Drawing for the job (mm, zero at the part's lowest x, y, z). Give positions to 0.01 mm unless a question says otherwise; leave off trailing zeros.
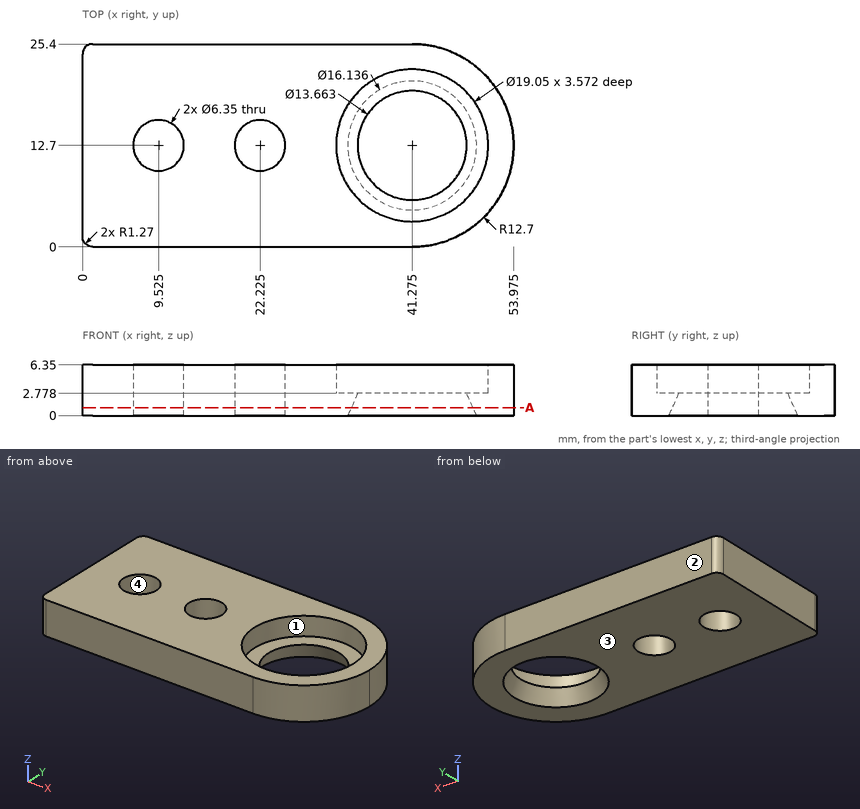
1. Pull direction Y, two halves, no side cores. Call the marked faces 1, 2, 3 and 4: +Y half, -Y half, draft (parallel to the pull), parting line (faces both ways), or undercut.
Calculated:
face 1: undercut
face 2: +Y half
face 3: draft
face 4: undercut
2. Slice it at A-A, the plane z = 1. State how many separate pieces and enclosed holes the cut face has, and give its area (4 significant figures).
Calculated:
separate pieces: 1
enclosed holes: 3
area: 1,055 mm2
3. Pin check, flat tips, straight feed: P1, Ø3, axis at x = 43.5, z = 2.5, coming from the +Y side; P2, Ø4, axis at x = 22.225, y = 12.7, coming from the -Z side. Stop position of each tip, or through.
Calculated:
P1: stops at y = 25.38
P2: passes through
4. Probe probe 1 along X at (y, z) = (13, 5) (1 decimal); probe 2 along Y at (x, z) = (41, 5.5); probe 3 along X at (y, z) = (13.5, 1.5). List the from-to ranges inside material, lowest first.
Calculated:
probe 1: x = 0 to 6.4, 12.7 to 19.1, 25.4 to 31.8, 50.8 to 54
probe 2: y = 0 to 3.18, 22.22 to 25.4
probe 3: x = 0 to 6.45, 12.6 to 19.15, 25.3 to 33.92, 48.63 to 53.95
